Check sheet for the modelled part. Datum: model origin and axes. Units: mm. Face numbers are marked on the shaded views. A direction names the side the tool comes from. Coordinates: 2 decimals unless noted, no trailing zeros. Loops run counter-clockwise (first coordinate to the right, second up) from the corner with the lowest first, then second, coordinate; pieces in that order, holes last. Notation, with made-up numbers: (36, -17) - (80, -17) arc R23 cw to (80, 5) - close; hole circle Ø6 at (-38.75, 9.25). An arc over 180 degrees is marked (long way). Answer as a JSON object with one key per item and string values. Group by question number.
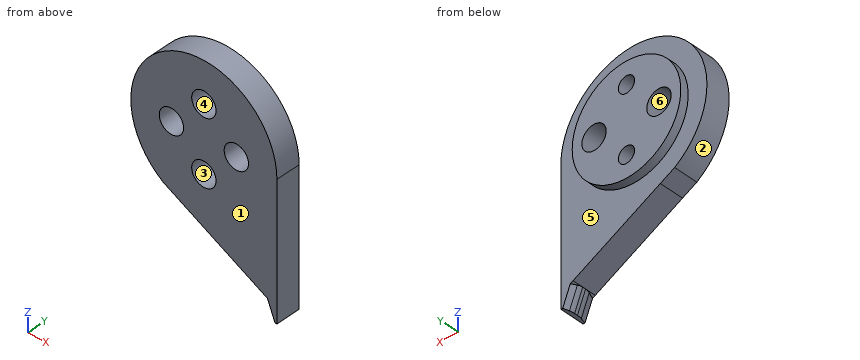
from build123d import *

# Parameters (mm, degrees)
F1_DEPTH    = 6
F2_SIZE2    = 4.99999
F2_SIZE     = 1.99999
F3_T4_DEPTH = 15.7736618076
F3_T9_DEPTH = 15.7736618076
F4_T4_DEPTH = 8.4627924491
F4_T9_DEPTH = 8.4627924491
F5_R        = 13.3817573781
F5_R_2      = 3
F5_R_3      = 2
F6_DEPTH    = 8
F7_DEPTH    = 8.001
F8_DEPTH    = 5


# Not quite as in the source:
# - a fillet or chamfer that OpenCascade refuses, or shapes differently, is made with other operations: its cross-section is extruded or revolved along the edge and cut away or added
# - a fillet or chamfer is up to 0.001 mm smaller than in the source, because OpenCascade refuses the exact size


with BuildPart() as f1:
    # F0 (on Front) → F1 (new body)
    with BuildSketch(Plane.XZ):
        with BuildLine():
            ThreePointArc((-6.5061441265, -16.7830297803), (10.1707769055, -14.8511042397), (18, 0))
            ThreePointArc((18, 0), (-8.4642142433, 15.8857507611), (-10.0396752493, -14.9400442064))
            Line((-10.0396752493, -14.9400442064), (-6.5061441265, -16.7830297803))
        make_face()
        with BuildLine():
            Line((18, -33), (18, 0))
            ThreePointArc((18, 0), (10.1707769055, -14.8511042397), (-6.5061441265, -16.7830297803))
            Line((-6.5061441265, -16.7830297803), (15, -28))
            Line((15, -28), (15, -33))
            Line((15, -33), (18, -33))
        make_face()
    extrude(amount=F1_DEPTH)

    # F2 (size 2 and 5 in the source; OpenCascade refuses exactly that, so slightly less here)
    f2_edges = [f1.edges().sort_by_distance(p)[0] for p in [
        (15, -3, -33),
    ]]
    f2_side = f1.faces().sort_by_distance((16.5, -3, -33))[0]
    chamfer(f2_edges, length=F2_SIZE, length2=F2_SIZE2, reference=f2_side)

    # F3: chamfer of 0.5 x 2 on 2 edges, made by hand


with BuildPart() as f3_tool2:
    # F3_s3 → F3_t4 (new body)
    with BuildSketch(Plane(origin=(15.653192591, 0, -39.1330988771), x_dir=(0, 1, 0), z_dir=(-0.3713897159, 0, 0.9284770751))):
        Polygon((0, -4.0282403683), (-2, -3.5282403683), (0, -3.5282403683), align=None)
    extrude(amount=F3_T4_DEPTH)

    split(bisect_by=Plane(origin=(-8.2729096879, 0, -15.8615369933), x_dir=(0, 1, 0), z_dir=(-0.4624484745, 0, -0.8866461574)), keep=Keep.TOP)


with BuildPart() as f1_1:
    add(f1.part)

    # F3_t1: cut F3_tool2
    add(f3_tool2.part, mode=Mode.SUBTRACT)


with BuildPart() as f3_tool7:
    # F3_s8 → F3_t9 (new body)
    with BuildSketch(Plane(origin=(15.653192591, 0, -39.1330988771), x_dir=(0, 1, 0), z_dir=(-0.3713897159, 0, 0.9284770751))):
        Polygon((-4, -3.5282403683), (-6, -4.0282403683), (-6, -3.5282403683), align=None)
    extrude(amount=F3_T9_DEPTH)

    split(bisect_by=Plane(origin=(-8.2729096879, 0, -15.8615369933), x_dir=(0, 1, 0), z_dir=(-0.4624484745, 0, -0.8866461574)), keep=Keep.TOP)


with BuildPart() as f1_2:
    add(f1_1.part)

    # F3_t6: cut F3_tool7
    add(f3_tool7.part, mode=Mode.SUBTRACT)

    # F4: fillet of radius 5 on 2 edges, made by hand


with BuildPart() as f4_tool2:
    # F4_s3 → F4_t4 (new body)
    with BuildSketch(Plane(origin=(14.2956017442, 0, -35.739111578), x_dir=(0, 1, 0), z_dir=(-0.3713897159, 0, 0.9284770751))):
        with BuildLine():
            ThreePointArc((-1.4028500029, -3.6775278676), (-2.0046118096, -3.5657025849), (-2.615528128, -3.5282403683))
            Line((-2.615528128, -3.5282403683), (-2, -3.5282403683))
            Line((-2, -3.5282403683), (-1.4028500029, -3.6775278676))
        make_face()
    extrude(amount=F4_T4_DEPTH)

    split(bisect_by=Plane(origin=(-8.2729096879, 0, -15.8615369933), x_dir=(0, 1, 0), z_dir=(-0.4624484745, 0, -0.8866461574)), keep=Keep.TOP)


with BuildPart() as f1_3:
    add(f1_2.part)

    # F4_t1: cut F4_tool2
    add(f4_tool2.part, mode=Mode.SUBTRACT)


with BuildPart() as f4_tool7:
    # F4_s8 → F4_t9 (new body)
    with BuildSketch(Plane(origin=(14.2956017442, 0, -35.739111578), x_dir=(0, 1, 0), z_dir=(-0.3713897159, 0, 0.9284770751))):
        with BuildLine():
            ThreePointArc((-4.5971499971, -3.6775278676), (-3.9953881904, -3.5657025849), (-3.384471872, -3.5282403683))
            Line((-3.384471872, -3.5282403683), (-4, -3.5282403683))
            Line((-4, -3.5282403683), (-4.5971499971, -3.6775278676))
        make_face()
    extrude(amount=F4_T9_DEPTH)

    split(bisect_by=Plane(origin=(-8.2729096879, 0, -15.8615369933), x_dir=(0, 1, 0), z_dir=(-0.4624484745, 0, -0.8866461574)), keep=Keep.TOP)


with BuildPart() as f1_4:
    add(f1_3.part)

    # F4_t6: cut F4_tool7
    add(f4_tool7.part, mode=Mode.SUBTRACT)

    # F5 (on face) → F6 (join)
    with BuildSketch(Plane.XZ.offset(6)):
        Circle(F5_R)
        with Locations((0, -8)):
            Circle(F5_R_2, mode=Mode.SUBTRACT)
        with Locations((-8, 0)):
            Circle(F5_R_2, mode=Mode.SUBTRACT)
        with Locations((8, 0)):
            Circle(F5_R_2, mode=Mode.SUBTRACT)
        with Locations((0, 8)):
            Circle(F5_R_2, mode=Mode.SUBTRACT)
        with Locations((0, 8)):
            Circle(F5_R_2)
        with Locations((0, 8)):
            Circle(F5_R_3, mode=Mode.SUBTRACT)
        with Locations((0, -8)):
            Circle(F5_R_2)
        with Locations((0, -8)):
            Circle(F5_R_3, mode=Mode.SUBTRACT)
        with Locations((-8, 0)):
            Circle(F5_R_2)
        with Locations((8, 0)):
            Circle(F5_R_2)
        with Locations((0, 8)):
            Circle(F5_R_3)
        with Locations((0, -8)):
            Circle(F5_R_3)
    extrude(amount=-F6_DEPTH)

    # F5 (on face) → F7 (cut, through all)
    with BuildSketch(Plane.XZ.offset(6)):
        with Locations((-8, 0)):
            Circle(F5_R_2)
        with Locations((0, 8)):
            Circle(F5_R_3)
        with Locations((8, 0)):
            Circle(F5_R_2)
        with Locations((0, -8)):
            Circle(F5_R_3)
    extrude(amount=-F7_DEPTH, mode=Mode.SUBTRACT)

    # F5 (on face) → F8 (cut)
    with BuildSketch(Plane.XZ.offset(6)):
        with Locations((0, 8)):
            Circle(F5_R_2)
        with Locations((0, 8)):
            Circle(F5_R_3, mode=Mode.SUBTRACT)
        with Locations((0, -8)):
            Circle(F5_R_2)
        with Locations((0, -8)):
            Circle(F5_R_3, mode=Mode.SUBTRACT)
    extrude(amount=-F8_DEPTH, mode=Mode.SUBTRACT)


solid = f1_4.part
1. Sectioned sample at C-C on y = 1. Record the cut outline in (x, z), plus the area to 3 significant figures.
2. Gauge pin test, flat ends, axial feed: pin 1 (5 mm diameter, centred on x = -1.5, z = -9.5, fed in from -Y); pin 2 (4 mm diameter, centred on x = 13.5, y = -4.5, fed in from +Z); pin 3 (4 mm diameter, centred on y = -4.5, z = -16.5, fed in from -X); pin 4 (1.5 mm diameter, centred on x = -11.5, y = -1, fed in from +Z). Record the tip position at first contact, or that the pin passes through.
3. Sectioned sample at A-A on x = -8. Record the cut outline in (y, z).
4. Access from +Z, -Z, +X, -X, +Y, -Y to the whole of each face (thin tool, end or side, straight path). Record for the marked faces 4, 5 and 6.
5. Sectioned sample at B-B on z = -7. Record the cut outline in (x, y).
6. Material ranges on line 1 (Z direction, x = 0, y = 0.2); line 2 (X direction, y = -4, z = -0.5); line 3 (Z direction, x = 0, y = -5), recorded low to high.
7. Sectioned sample at D-D on x = 0. Record the cut outline in (y, z).
8. Release check for a two-part mould opening along X. For the marked faces 1, 2 and 3 record: released by +X, released by -X, zero draft, split by the parting line, or undercut.
Answers follow:
{
 "1": {"outline": "circle Ø26.76 at (0, 0); hole circle Ø6 at (-8, 0); hole circle Ø4 at (0, -8); hole circle Ø4 at (0, 8); hole circle Ø6 at (8, 0)", "area": "481 mm^2"},
 "2": {"pin 1": "stops at y = -6", "pin 2": "stops at z = 13.85", "pin 3": "stops at x = -10.67", "pin 4": "stops at z = 14.44"},
 "3": {"outline": "(-6, -16) - (0, -16) - (0, -10.73) - (2, -10.73) - (2, -3) - (-6, -3) - close; (-6, 3) - (2, 3) - (2, 10.73) - (0, 10.73) - (0, 16.12) - (-6, 16.12) - close"},
 "4": {"face 4": "-Y", "face 5": "+Y", "face 6": "+Y, -Y"},
 "5": {"outline": "(-16.58, -6) - (-2.83, -6) - (-2.83, -1) - (-1.73, -1) - (-1.73, 2) - (-11.4, 2) - (-11.4, 0) - (-16.58, 0) - close; (1.73, -1) - (2.83, -1) - (2.83, -6) - (18, -6) - (18, 0) - (11.4, 0) - (11.4, 2) - (1.73, 2) - close"},
 "6": {"line 1": "z = -13.38 to -10, -6 to 6, 10 to 13.38", "line 2": "x = -17.99 to -10.96, -5.04 to 5.04, 10.96 to 18", "line 3": "z = -20.18 to -11, -5 to 5, 11 to 18"},
 "7": {"outline": "(-6, -20.18) - (0, -20.18) - (0, -13.38) - (2, -13.38) - (2, -10) - (-1, -10) - (-1, -11) - (-6, -11) - close; (-6, -5) - (-1, -5) - (-1, -6) - (2, -6) - (2, 6) - (-1, 6) - (-1, 5) - (-6, 5) - close; (-6, 11) - (-1, 11) - (-1, 10) - (2, 10) - (2, 13.38) - (0, 13.38) - (0, 18) - (-6, 18) - close"},
 "8": {"face 1": "zero draft", "face 2": "split by the parting line", "face 3": "undercut"}
}
